Geometry: final body of the model. Coordinates: model frame, mm. A direction names the side the tool comes from. Give positions to 0.01 mm unless a question says otherwise; leave off trailing zeros. Write each loop counter-clockwise with the first axis right and the second up, starting at its lowest first coordinate (ties: lowest second). Pieces come first, ordered by that corner, then holes. Notation, with made-up numbers: M 18.5,86 L 62.5,86 A7 cw 62.5,91 Z; hole C 22,40.5 d3. An arc over 180 degrees is marked long. Answer as a JSON object with one key per item and string values.
from build123d import *

# Parameters (mm, degrees)
SKETCH1_R           = 26
SKETCH1_R_2         = 20.875
BOSS_EXTRUDE1_DEPTH = 7.5
SKETCH2_R           = 5.25
SKETCH3_W           = 1
SKETCH3_H           = 0.625
FILLET1_R           = 1


with BuildPart() as part:
    # Sketch1 → Boss-Extrude1 (new, symmetric)
    with BuildSketch(Plane(origin=(0, 0, 0), x_dir=(0, 0, -1), z_dir=(1, 0, 0))):
        Circle(SKETCH1_R)
        Circle(SKETCH1_R_2, mode=Mode.SUBTRACT)
    extrude(amount=BOSS_EXTRUDE1_DEPTH, both=True)

    # Sketch2 → Cut-Revolve1 (revolve, cut)
    with BuildSketch(Plane.XY, mode=Mode.PRIVATE) as cut_revolve1_sk:
        with Locations((0, 17.5)):
            Circle(SKETCH2_R)
    revolve(cut_revolve1_sk.sketch.rotate(Axis((0, 0, 0), (1, 0, 0)), 90), axis=Axis((0, 0, 0), (1, 0, 0)), mode=Mode.SUBTRACT)

    # Sketch3 → Cut-Revolve2 (revolve, cut)
    with BuildSketch(Plane.XY, mode=Mode.PRIVATE) as cut_revolve2_sk:
        with Locations((-6.5, 21.1875)):
            Rectangle(SKETCH3_W, SKETCH3_H)
        with Locations((6.5, 21.1875)):
            Rectangle(SKETCH3_W, SKETCH3_H)
    revolve(cut_revolve2_sk.sketch.rotate(Axis((0, 0, 0), (1, 0, 0)), 90), axis=Axis((0, 0, 0), (1, 0, 0)), mode=Mode.SUBTRACT)

    # Fillet1
    fillet1_edges = [part.edges().sort_by_distance(p)[0] for p in [
        (-7.5, 0, 26),
        (7.5, 0, 26),
    ]]
    fillet(fillet1_edges, radius=FILLET1_R)


solid = part.part
1) Set-up query: faces 5 (the flat face through (-7.5, -20.3, 5.7)), 6 (the cylindrical face through (-6.493, -21.317, -2.799)). Return all of +Z, -Z, +X, -X, +Y, -Y with unobstructed straight access to the full face (end or side cutting, diameter ignored); none if empty.
Geometry check:
{"face 5": "+Z, -Z, -X, +Y, -Y", "face 6": "none"}
2) Pull-direction query (Z, two-part tool) for faces 1 (the flat face through (7.5, -20.3, 5.7)), 2 (the cylindrical face through (6.507, -21.317, -2.799)), 3 (the cylindrical face through (0.091, -15.821, 20.633)), 4 (the flat face through (-7, -11, 18)); classes: pulls with the +Z half, pulls with the -Z half, needs draft (parallel to the pull), parting line crosses it, or undercut.
Geometry check:
{"face 1": "needs draft", "face 2": "undercut", "face 3": "parting line crosses it", "face 4": "undercut"}
3) Cut plane C-C on x = 3. Return loops of the section in (y, z).
Geometry check:
{"outline": "C 0,0 d52; hole C 0,0 d43.62"}
4) Contact query for flat-ended pins moving along their axis: P1, Ø1, axis at x = -3.5, z = -9.5, coming from the +Y side; P2, Ø13, axis at y = -7.5, z = 6, coming from the +X side; P3, Ø2, axis at x = -1.5, z = 18.5, coming from the +Y side; P4, Ø6, axis at x = -4, y = -15, coming from the -Z side. Output: stop coordinate, or through.
Geometry check:
{"P1": "stops at y = 24.39", "P2": "passes through", "P3": "stops at y = 19.23", "P4": "stops at z = -23.07"}
5) Line query: line 1 (Y direction, x = 4.7, z = 0) (3 decimals); line 2 (Y direction, x = 6.55, z = 0); line 3 (Z direction, x = 7.25, y = -0.5). Output: solid intervals per line, ascending. Write a range as from..to.
Geometry check:
{"line 1": "y = -26..-20.875, 20.875..26", "line 2": "y = -26..-21.5, 21.5..26", "line 3": "z = -25.66..-20.87, 20.87..25.66"}
